Verification items for the finished model (mm, model axes). Face numbers are marked on the shaded views. A direction names the side the tool comes from. Round coordinates to 2 decimals unless told otherwise and drop trailing zeros. Order: outer loops, then holes, each group sorted by start corner. A loop starts at its lowest first (then second) coordinate and runs counter-clockwise, first axis right, second up. Notation, with made-up numbers: (15.5, 64.25) -> (56.5, 64.25) arc R23 ccw to (56.5, 91.25) -> close; hole circle Ø9 at (31, 71.25). An arc over 180 degrees is marked (long way). Return JSON: item names as keys, results as strings. Group by question number.
1) Section check A-A on x = -8.75. Enter the section's corners in (y, z) (3 decimals), plus the area to 4 significant figures.
2) Section check D-D on z = 34.5. Enter the section's corners in (x, y), plus the area to 3 significant figures.
3) Draft check along Z on the marked faces 1, 2 and 3. Enter one of: pulls with the +Z half, pulls with the -Z half, needs draft (parallel to the pull), parting line crosses it, or undercut.
4) Section check B-B on y = -32. State how many separate pieces and enclosed holes the cut face has, plus the area to 3 significant figures.
5) Scan lines: L1, parallel to X at y = -31.75, z = 50; L2, parallel to X at y = -27.56, z = 8.45; L3, parallel to Z at x = -6, y = -29. Record each from-to range of solid material in increasing order.
6) Depth check by flat-ended pin: pin 1 (9 mm diameter, centred on y = -30, z = 29, fed in from -X); pin 2 (5 mm diameter, centred on x = -10.5, z = 52.5, fed in from +Y); pin 3 (4 mm diameter, centred on x = -9.5, z = 48, fed in from -Y). Enter the tip coordinate at first touch or a pass-through.
7) Section check C-C on x = 17. Enter the section's corners in (y, z), plus the area to 3 significant figures.
8) Tool access check on the marked faces 4, 5 and 6. Record the directions out of +Z, -Z, +X, -X, +Y, -Y that give a thin tool (end or side, any length) a straight path to the whole face; none if there is none.
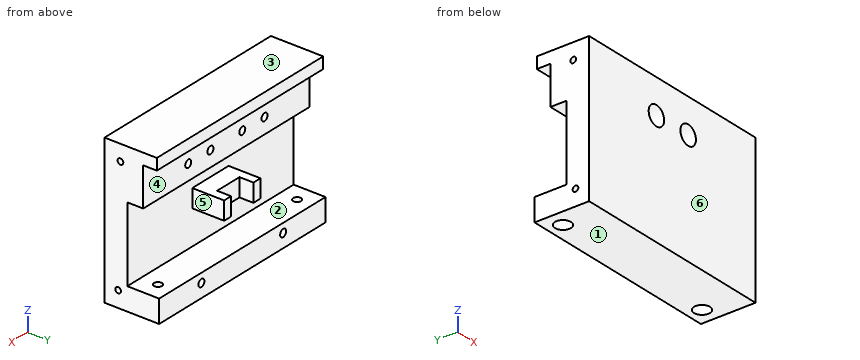
```python
from build123d import *

# Parameters (mm, degrees)
SKETCH1_W                  = 91.58
SKETCH1_H                  = 70.12
SKETCH1_R                  = 1.75
BOSS_EXTRUDE1_DEPTH        = 10
SKETCH2_W                  = 91.58
SKETCH2_H                  = 65
BOSS_EXTRUDE2_DEPTH        = 10
SKETCH3_W                  = 20
SKETCH3_H                  = 8
BOSS_EXTRUDE3_DEPTH        = 14
CUT_EXTRUDE1_DEPTH         = 75
SKETCH6_W                  = 91.58
SKETCH6_H                  = 65
CUT_EXTRUDE3_DEPTH         = 98.319979963
SKETCH11_W                 = 91.58
SKETCH11_H                 = 22
BOSS_EXTRUDE4_DEPTH        = 7
SKETCH12_W                 = 91.58
SKETCH12_H                 = 5
BOSS_EXTRUDE5_DEPTH        = 6
M4_TAPPED_HOLE2_D          = 3.3
M4_TAPPED_HOLE2_DEPTH      = 10
M4_TAPPED_HOLE2_TIP        = 0.991420021
SKETCH16_R                 = 4.25
CUT_EXTRUDE4_DEPTH         = 12
M4_TAPPED_HOLE3_D          = 3.3
SKETCH21_R                 = 3.5
CUT_EXTRUDE5_DEPTH         = 4
M4_TAPPED_HOLE4_D          = 3.3
M4_TAPPED_HOLE4_DEPTH      = 15
M4_TAPPED_HOLE4_TIP        = 0.991420021
M3_TAPPED_HOLE1_AT_2_COUNT = 2
M3_TAPPED_HOLE1_AT_2_PITCH = 51.009802979


with BuildPart() as part:
    # Sketch1 → Boss-Extrude1 (new body)
    with BuildSketch(Plane.XY):
        Rectangle(SKETCH1_W, SKETCH1_H)
        with Locations((-16.825414035, 27.05)):
            Circle(SKETCH1_R, mode=Mode.SUBTRACT)
        with Locations((33.464, 27.56)):
            Circle(SKETCH1_R, mode=Mode.SUBTRACT)
        with Locations((38.29, -27.56)):
            Circle(SKETCH1_R, mode=Mode.SUBTRACT)
        with Locations((-38.29, -27.56)):
            Circle(SKETCH1_R, mode=Mode.SUBTRACT)
    extrude(amount=BOSS_EXTRUDE1_DEPTH)

    # Sketch2 → Boss-Extrude2 (add)
    with BuildSketch(Plane.XZ.offset(35.06)):
        with Locations((0, 32.5)):
            Rectangle(SKETCH2_W, SKETCH2_H)
    extrude(amount=BOSS_EXTRUDE2_DEPTH)

    # Sketch3 → Boss-Extrude3 (add)
    with BuildSketch(Plane(origin=(0, -35.06, 0), x_dir=(1, 0, 0), z_dir=(0, 1, 0))):
        with Locations((0, -29)):
            Rectangle(SKETCH3_W, SKETCH3_H)
    extrude(amount=BOSS_EXTRUDE3_DEPTH)

    # Sketch4 → Cut-Extrude1 (cut)
    with BuildSketch(Plane(origin=(0, 0, 25), x_dir=(-1, 0, 0), z_dir=(0, 0, -1))):
        Polygon((6.15, -21.06), (6.15, -14.91), (-6.15, -14.91), (-6.15, -21.06), (-6.15, -27.21), (6.15, -27.21), align=None)
    extrude(amount=-CUT_EXTRUDE1_DEPTH, mode=Mode.SUBTRACT)

    # Sketch6 → Cut-Extrude3 (cut, through all)
    with BuildSketch(Plane(origin=(0, -21.06, 0), x_dir=(1, 0, 0), z_dir=(0, 1, 0))):
        with Locations((0, -32.5)):
            Rectangle(SKETCH6_W, SKETCH6_H)
    extrude(amount=CUT_EXTRUDE3_DEPTH, mode=Mode.SUBTRACT)

    # Sketch11 → Boss-Extrude4 (add)
    with BuildSketch(Plane(origin=(0, -35.06, 0), x_dir=(1, 0, 0), z_dir=(0, 1, 0))):
        with Locations((0, -54)):
            Rectangle(SKETCH11_W, SKETCH11_H)
    extrude(amount=BOSS_EXTRUDE4_DEPTH)

    # Sketch12 → Boss-Extrude5 (add)
    with BuildSketch(Plane(origin=(0, -28.06, 0), x_dir=(1, 0, 0), z_dir=(0, 1, 0))):
        with Locations((0, -62.5)):
            Rectangle(SKETCH12_W, SKETCH12_H)
    extrude(amount=BOSS_EXTRUDE5_DEPTH)

    # M4 Tapped Hole2
    with Locations(Plane(origin=(0, -28.06, 0), x_dir=(1, 0, 0), z_dir=(0, 1, 0))):
        with Locations((21, -49.825), (-21, -49.825)):
            Hole(M4_TAPPED_HOLE2_D / 2, depth=M4_TAPPED_HOLE2_DEPTH)
            with Locations((0, 0, -(M4_TAPPED_HOLE2_DEPTH + M4_TAPPED_HOLE2_TIP / 2))):  # 118° drill point
                Cone(0, M4_TAPPED_HOLE2_D / 2, M4_TAPPED_HOLE2_TIP, mode=Mode.SUBTRACT)

    # Sketch16 → Cut-Extrude4 (cut)
    with BuildSketch(Plane.XZ.offset(45.06)):
        with Locations(Location((-8.75, 49.825, 0), (0, 0, 270))):
            Circle(SKETCH16_R)
        with Locations(Location((8.75, 49.825, 0), (0, 0, 270))):
            Circle(SKETCH16_R)
    extrude(amount=-CUT_EXTRUDE4_DEPTH, mode=Mode.SUBTRACT)

    # M4 Tapped Hole3 (through all)
    with Locations(Plane(origin=(0, -33.06, 0), x_dir=(-1, 0, 0), z_dir=(0, -1, 0))):
        with Locations((8.75, -49.825), (-8.75, -49.825)):
            Hole(M4_TAPPED_HOLE3_D / 2)

    # Sketch21 → Cut-Extrude5 (cut)
    with BuildSketch(Plane(origin=(0, 0, 0), x_dir=(-1, 0, 0), z_dir=(0, 0, -1))):
        with Locations((-38.29, -27.56)):
            Circle(SKETCH21_R)
        with Locations((38.29, -27.56)):
            Circle(SKETCH21_R)
    extrude(amount=-CUT_EXTRUDE5_DEPTH, mode=Mode.SUBTRACT)

    # M4 Tapped Hole4
    with Locations(Plane(origin=(0, -21.06, 0), x_dir=(1, 0, 0), z_dir=(0, 1, 0))):
        with Locations((-22.5, -6), (22.5, -6)):
            Hole(M4_TAPPED_HOLE4_D / 2, depth=M4_TAPPED_HOLE4_DEPTH)
            with Locations((0, 0, -(M4_TAPPED_HOLE4_DEPTH + M4_TAPPED_HOLE4_TIP / 2))):  # 118° drill point
                Cone(0, M4_TAPPED_HOLE4_D / 2, M4_TAPPED_HOLE4_TIP, mode=Mode.SUBTRACT)

    # Sketch27 → M3 Tapped Hole1 (revolve, cut)
    with BuildSketch(Plane(origin=(-45.79, -38.06, 58), x_dir=(0, 0, 1), z_dir=(0, 1, 0))):
        Polygon((0, 0), (0, 8.251075774), (1.25, 7.5), (1.25, 0), align=None)
    m3_tapped_hole1 = revolve(axis=Axis((-52.14, -38.06, 58), (1, 0, 0)), mode=Mode.SUBTRACT)

    # M3 Tapped Hole1 at 2: M3 Tapped Hole1 ×2
    with Locations(*[Vector(0, -0.0196040749344456, -0.9998078216567245) * (i * M3_TAPPED_HOLE1_AT_2_PITCH) for i in range(1, M3_TAPPED_HOLE1_AT_2_COUNT)]):
        add(m3_tapped_hole1, mode=Mode.SUBTRACT)

    # Mirror1: M3 Tapped Hole1 across plane
    add(m3_tapped_hole1.mirror(Plane(origin=(0, 0, 0), x_dir=(0, 0, 1), z_dir=(1, 0, 0))), mode=Mode.SUBTRACT)

    # Mirror1 copy 1 sketch → Mirror1 copy 1 (revolve, cut)
    with BuildSketch(Plane(origin=(45.79, -39.06, 7), x_dir=(0, 0, 1), z_dir=(0, 1, 0))):
        Polygon((0, 0), (0, -8.251075774), (1.25, -7.5), (1.25, 0), align=None)
    revolve(axis=Axis((52.14, -39.06, 7), (1, 0, 0)), mode=Mode.SUBTRACT)


solid = part.part
```
Check result:
{
 "1": {"outline": "(-45.06, 0) -> (-21.06, 0) -> (-21.06, 10) -> (-35.06, 10) -> (-35.06, 25) -> (-21.06, 25) -> (-21.06, 33) -> (-35.06, 33) -> (-35.06, 43) -> (-28.06, 43) -> (-28.06, 48.175) -> (-33.06, 48.175) -> (-33.06, 45.575) -> (-45.06, 45.575) -> close; (-45.06, 54.075) -> (-33.06, 54.075) -> (-33.06, 51.475) -> (-28.06, 51.475) -> (-28.06, 60) -> (-22.06, 60) -> (-22.06, 65) -> (-45.06, 65) -> close", "area": "967.5 mm^2"},
 "2": {"outline": "(-45.79, -45.06) -> (45.79, -45.06) -> (45.79, -35.06) -> (-45.79, -35.06) -> close", "area": "916 mm^2"},
 "3": {"face 1": "pulls with the -Z half", "face 2": "undercut", "face 3": "pulls with the +Z half"},
 "4": {"separate pieces": "3", "enclosed holes": "6", "area": "3,040 mm^2"},
 "5": {"L1": "-45.79 to -22.64, -19.36 to -10.39, -7.11 to 7.11, 10.39 to 19.36, 22.64 to 45.79", "L2": "-45.79 to -40.04, -36.54 to 36.54, 40.04 to 45.79", "L3": "0 to 10, 25 to 33, 43 to 65"},
 "6": {"pin 1": "x = -10", "pin 2": "y = -28.06", "pin 3": "y = -33.06"},
 "7": {"outline": "(-45.06, 0) -> (-21.06, 0) -> (-21.06, 10) -> (-35.06, 10) -> (-35.06, 43) -> (-28.06, 43) -> (-28.06, 60) -> (-22.06, 60) -> (-22.06, 65) -> (-45.06, 65) -> close", "area": "974 mm^2"},
 "8": {"face 4": "+X, -X, +Y", "face 5": "+X, +Y", "face 6": "+Z, -Z, +X, -X, -Y"}
}
